```python
from build123d import *

# Parameters (mm, degrees)
F0_W     = 50.8
F0_H     = 38.1
F1_DEPTH = 12.7
F2_W     = 17.091405
F2_H     = 15.964834
F3_DEPTH = 12.701
F4_W     = 50.8
F4_H     = 44.45
F5_DEPTH = 12.7
F7_DEPTH = 12.7
F8_R     = 12.7
F9_DEPTH = 12.701


with BuildPart() as f1:
    # F0 (on Front) → F1 (new body)
    with BuildSketch(Plane.XZ):
        Rectangle(F0_W, F0_H)
    extrude(amount=F1_DEPTH)

    # F2 (on Front) → F3 (cut, through all)
    with BuildSketch(Plane.XZ):
        with Locations((21.245703, 14.332417)):
            Rectangle(F2_W, F2_H)
    extrude(amount=F3_DEPTH, mode=Mode.SUBTRACT)

    # F4 (on face) → F5 (join)
    with BuildSketch(Plane(origin=(0, 0, -19.05), x_dir=(1, 0, 0), z_dir=(0, 0, -1))):
        with Locations((0, -22.225)):
            Rectangle(F4_W, F4_H)
    extrude(amount=-F5_DEPTH)

    # F6 (on face) → F7 (join)
    with BuildSketch(Plane.XY.offset(-6.35)):
        with BuildLine():
            Line((-25.4, 44.45), (25.4, 44.45))
            ThreePointArc((25.4, 44.45), (0, 69.85), (-25.4, 44.45))
        make_face()
    extrude(amount=-F7_DEPTH)

    # F8 (on face) → F9 (cut, through all)
    with BuildSketch(Plane.XY.offset(-6.35)):
        with Locations((0, 44.45)):
            Circle(F8_R)
    extrude(amount=-F9_DEPTH, mode=Mode.SUBTRACT)


solid = f1.part
```
Read the model definition and answer for the solid it produces. Units are mm, in the model's axes. A direction names the side the tool comes from. Coordinates: 2 decimals unless noted, no trailing zeros. Loops run counter-clockwise (first coordinate to the right, second up) from the corner with the lowest first, then second, coordinate; pieces in that order, holes last.
(1) The part is cut by section D-D (x = 20). Determine the outline of the cut face in (y, z), and give its area (3 significant figures).
Solution:
outline: (-12.7, -19.05) - (60.11, -19.05) - (60.11, -6.35) - (0, -6.35) - (0, 6.35) - (-12.7, 6.35) - close
area: 1,090 mm2
(2) The part is cut by section A-A (x = 0). Determine the outline of the cut face in (y, z).
Solution:
outline: (-12.7, -19.05) - (31.75, -19.05) - (31.75, -6.35) - (0, -6.35) - (0, 19.05) - (-12.7, 19.05) - close; (57.15, -19.05) - (69.85, -19.05) - (69.85, -6.35) - (57.15, -6.35) - close
(3) The mould has two halves that part along Y. Classify faces 4 (the face through (0, 20, -19.05)), 5 (the face through (0, -12.7, 0)), 6 (the face through (-2.75, 32.05, -12.61)): released by +Y, released by -Y, zero draft, split by the parting line, or undercut.
Solution:
face 4: zero draft
face 5: released by -Y
face 6: undercut
(4) A tool of negligible diameter and unlimited length cuts with its end or side. For faces 1 (the face through (12.7, -6, 13)), 2 (the face through (0.559, 69.844, -12.611)), 3 (the face through (0, 28, -6.35)), from which of +Z, -Z, +X, -X, +Y, -Y can it reach the whole face along a straight path? Write none if from no direction.
Solution:
face 1: +Z, +X, +Y, -Y
face 2: +Z, -Z, +Y
face 3: +Z, +X, -X, +Y
(5) Flat-ended cylindrical pins translate along their axes: pin 1 Ø8 at (x, y) = (-20, 23.5) entering from +Z; pin 2 Ø4 at (y, z) = (-7, 14.5) entering from +X; pin 3 Ø3 at (x, y) = (-0.5, 26.5) entering from +Z. Find the tip coordinate at first contact, or state that the pin passes through.
Solution:
pin 1: stops at z = -6.35
pin 2: stops at x = 12.7
pin 3: stops at z = -6.35
(6) Consider line 1 along Y through (x, z) = (0, -16); line 2 along X through (y, z) = (44, -12); line 3 along Y through (x, z) = (6, -3). Determine where each line is inside the solid, lowest interval first.
Solution:
line 1: y = -12.7 to 31.75, 57.15 to 69.85
line 2: x = -25.4 to -12.69, 12.69 to 25.4
line 3: y = -12.7 to 0
(7) The part is cut by section C-C (y = 25.5). Determine the outline of the cut face in (x, z).
Solution:
outline: (-25.4, -19.05) - (25.4, -19.05) - (25.4, -6.35) - (-25.4, -6.35) - close
(8) The part is cut by section B-B (z = -12). Determine the outline of the cut face in (x, y), and give its area (3 significant figures).
Solution:
outline: (-25.4, -12.7) - (25.4, -12.7) - (25.4, 44.45) arc R25.4 ccw to (-25.4, 44.45) - close; hole circle Ø25.4 at (0, 44.45)
area: 3,410 mm2
